```python
from build123d import *

# Parameters (mm, degrees)
EXTRUDE_1_DEPTH     = 10
EXTRUDE_3_DEPTH     = 40
FILLET_2_R          = 3
FILLET_3_R          = 3
SKETCH_13_R         = 4.75
CUT_EXTRUDE_3_DEPTH = 10


with BuildPart() as part:
    # 草图3 → 凸台-拉伸1 (new body)
    with BuildSketch(Plane.XY):
        Polygon((-100, -79.175359259), (-100, -119.175359259), (-60, -119.175359259), (-60, -114.175359259), (-95, -79.175359259), align=None)
    extrude(amount=-EXTRUDE_1_DEPTH)

    # 草图5 → 切除-放样1 section 0
    with BuildSketch(Plane.XY.offset(-6)):
        with BuildLine():
            Line((-96.08, -104.799041882), (-96.08, -98.821989002))
            Line((-96.08, -98.821989002), (-81.709132385, -81.695455893))
            Line((-81.709132385, -81.695455893), (-66.265676412, -94.654054104))
            Line((-66.265676412, -94.654054104), (-83.579668035, -115.288065824))
            Line((-83.579668035, -115.288065824), (-96.08, -104.799041882))
        make_face()
    # 草图8 → 切除-放样1 section 1
    with BuildSketch(Plane.XY):
        with BuildLine():
            Line((-94.58, -104.099580395), (-94.58, -99.367944353))
            Line((-94.58, -99.367944353), (-80.56006572, -82.659637307))
            Line((-80.56006572, -82.659637307), (-67.414743077, -93.68987269))
            Line((-67.414743077, -93.68987269), (-83.764553285, -113.174817744))
            Line((-83.764553285, -113.174817744), (-94.58, -104.099580395))
        make_face()
    loft(mode=Mode.SUBTRACT)

    # 草图9 → 凸台-拉伸3 (add)
    with BuildSketch(Plane(origin=(0, 0, -10), x_dir=(-1, 0, 0), z_dir=(0, 0, -1))):
        Polygon((95, -79.175359259), (95, -114.175359259), (60, -114.175359259), (60, -119.175359259), (100, -119.175359259), (100, -79.175359259), align=None)
    extrude(amount=EXTRUDE_3_DEPTH)

    # 镜向2: part across plane


with BuildPart() as part_1:
    add(part.part)
    add(part.part.mirror(Plane(origin=(0, 0, -50), x_dir=(1, 0, 0), z_dir=(0, 0, -1))))

    # 圆角2
    fillet_2_edges = [part_1.edges().sort_by_distance(p)[0] for p in [
        (-60, -116.675359259, -100),
        (-60, -116.675359259, 0),
        (-100, -99.175359259, -100),
        (-100, -99.175359259, 0),
        (-100, -79.175359259, -50),
        (-97.5, -79.175359259, 0),
    ]]
    fillet(fillet_2_edges, radius=FILLET_2_R)

    # 圆角3
    fillet_3_edges = [part_1.edges().sort_by_distance(p)[0] for p in [
        (-80, -119.175359259, -100),
        (-80, -119.175359259, 0),
        (-100, -119.175359259, -50),
        (-60, -119.175359259, -50),
        (-99.121320344, -119.175359259, -0.878679656),
        (-99.121320344, -119.175359259, -99.121320344),
        (-60.878679656, -119.175359259, -0.878679656),
        (-60.878679656, -119.175359259, -99.121320344),
    ]]
    fillet(fillet_3_edges, radius=FILLET_3_R)

    # 草图13 → 切除-拉伸3 (cut)
    with BuildSketch(Plane.ZY.offset(100)):
        with Locations((-50, -88.175359259)):
            Circle(SKETCH_13_R)
    extrude(amount=-CUT_EXTRUDE_3_DEPTH, mode=Mode.SUBTRACT)


solid = part_1.part
```
The model under review builds one solid part; all positions refer to its coordinate system, in mm. A direction names the side the tool comes from. Coordinates: 2 decimals unless noted, no trailing zeros. Order: outer loops, then holes, each group sorted by start corner. A loop starts at its lowest first (then second) coordinate and runs counter-clockwise, first axis right, second up. Notation, with made-up numbers: (2, 38) -> (38, 38) arc R27 ccw to (38, 58) -> close; hole circle Ø9 at (42, 50). An arc over 180 degrees is marked (long way). Answer in a Markdown table with one row per item. Add a question column.
Item 1: Machinability: for faces 1 (the flat face through (-78, -114.175, -51)), 2 (the cylindrical face through (-61.252, -114.751, -99.438)), which of the approach directions +Z, -Z, +X, -X, +Y, -Y give a long, thin tool a straight path to every point of the face, cutting with its end or side? Answer none if there is none.
Item 2: Mouldability with a two-part tool opening along Y and no side actions: class faces 3 (the flat face through (-96, -79.175, -52)), 4 (the cylindrical face through (-79.762, -118.273, -99.145)), 5 (the flat face through (-85, -101, -94)) as +Y half, -Y half, draft (parallel to the pull), parting line (faces both ways), or undercut.
Item 3: To check wall thickness, follow probe 1 along Z at (x, y) = (-86.5, -99.5); probe 2 along Y at (x, z) = (-96.65, -50); probe 3 along Z at (x, y) = (-92.5, -109.5). State the ranges of each line that lie inside material, in increasing order.
Item 4: We need section D-D on x = -70.5. Write out the cut boundary in (y, z).
Item 5: We need section C-C on z = -14. Write out the cut boundary in (x, y), plus the area to 3 significant figures.
Item 6: We need section A-A on z = -50. Write out the cut boundary in (x, y), plus the area to 3 significant figures.
Item 7: We need section B-B on y = -86. Write out the cut boundary in (x, z).
Item 8: Clearance check with flat-ended pins moving along their axes: pin 1 (3 mm diameter, centred on y = -108, z = -56.5, fed in from +X); pin 2 (17.5 mm diameter, centred on x = -69.5, y = -95.5, fed in from +Z); pin 3 (4 mm diameter, centred on x = -86.5, y = -106, fed in from +Z); pin 4 (3 mm diameter, centred on x = -65, z = -61.5, fed in from +Y). State where each tip first meets the part, or that it passes through.
Final values:
| question | item | result |
|---|---|---|
| 1 | face 1 | +X, +Y |
| 1 | face 2 | -Z, +X, +Y, -Y |
| 2 | face 3 | +Y half |
| 2 | face 4 | -Y half |
| 2 | face 5 | undercut |
| 3 | probe 1 | z = -94 to -90, -10 to -6 |
| 3 | probe 2 | y = -119.18 to -92.93, -83.43 to -79.18 |
| 3 | probe 3 | z = -100 to -90, -10 to 0 |
| 4 | outline | (-119.18, -97) arc R3 ccw to (-116.18, -100) -> (-103.68, -100) -> (-103.68, -90) -> (-114.18, -90) -> (-114.18, -10) -> (-103.68, -10) -> (-103.68, 0) -> (-116.18, 0) arc R3 ccw to (-119.18, -3) -> close |
| 5 | outline | (-100, -116.18) arc R3 ccw to (-97, -119.18) -> (-63, -119.18) arc R3 ccw to (-60, -116.18) -> (-60, -114.18) -> (-95, -114.18) -> (-95, -79.18) -> (-97, -79.18) arc R3 ccw to (-100, -82.18) -> close |
| 5 | area | 369 mm2 |
| 6 | outline | (-100, -116.18) arc R3 ccw to (-97, -119.18) -> (-63, -119.18) arc R3 ccw to (-60, -116.18) -> (-60, -114.18) -> (-95, -114.18) -> (-95, -92.93) -> (-100, -92.93) -> close; (-100, -83.43) -> (-95, -83.43) -> (-95, -79.18) -> (-97, -79.18) arc R3 ccw to (-100, -82.18) -> close |
| 6 | area | 322 mm2 |
| 7 | outline | (-100, -97) arc R3 ccw to (-97, -100) -> (-88.18, -100) -> (-88.18, -90) -> (-95, -90) -> (-95, -54.22) -> (-100, -54.22) -> close; (-100, -45.78) -> (-95, -45.78) -> (-95, -10) -> (-88.18, -10) -> (-88.18, 0) -> (-97, 0) arc R3 ccw to (-100, -3) -> close |
| 8 | pin 1 | stops at x = -95 |
| 8 | pin 2 | stops at z = 0 |
| 8 | pin 3 | stops at z = -6 |
| 8 | pin 4 | stops at y = -114.18 |
